Verification items for the finished model (mm, model axes). A direction names the side the tool comes from. Round coordinates to 2 decimals unless told otherwise and drop trailing zeros. Order: outer loops, then holes, each group sorted by start corner. A loop starts at its lowest first (then second) coordinate and runs counter-clockwise, first axis right, second up. Notation, with made-up numbers: (70.5, 73) -> (99.5, 73) arc R26 ccw to (99.5, 95) -> close; hole circle Ø8 at (-2, -28.5). An arc over 180 degrees is marked (long way). Return JSON: item names as keys, results as strings. Group by question number.
1) Section check C-C on x = 0. Enter the section's corners in (y, z).
2) Section check A-A on y = 0. Enter the section's corners in (x, z), plus the area to 3 significant figures.
3) Depth check by flat-ended pin: pin 1 (0.7 mm diameter, centred on x = 0, y = 1, fed in from -Z); pin 2 (0.5 mm diameter, centred on y = 0.5, z = 0.5, fed in from +X). Enter the tip coordinate at first touch or a pass-through.
4) Section check B-B on z = 1.2. Enter the section's corners in (x, y), plus the area to 3 significant figures.
5) Section check D-D on z = 3.95. Enter the section's corners in (x, y).
6) Scan lines: L1, parallel to Y at x = -1.4, z = 1.45; L2, parallel to Y at x = -0.45, z = 2.7; L3, parallel to X at y = -0.4, z = 0.6. Record each from-to range of solid material in increasing order.
7) Tool access check on faces 4 (the flat face through (-0.444, 0, 1)), 5 (the flat face through (1, 0, 0)). Record the directions out of +Z, -Z, +X, -X, +Y, -Y that give a thin tool (end or side, any length) a straight path to the whole face; none if there is none.
8) Draft check along X on faces 1 (the cylindrical face through (1.008, -1.938, 2.317)), 2 (the flat face through (-1, 0, 0)), 3 (the flat face through (0, 0, 1.524)). Enter one of: pulls with the +X half, pulls with the -X half, needs draft (parallel to the pull), parting line crosses it, or undercut.
```python
from build123d import *

# Parameters (mm, degrees)
F0_R     = 2.1844
F1_DEPTH = 5.207
F2_W     = 0.889
F2_H     = 3.048
F3_DEPTH = 12.7
F4_SIZE  = 0.508


with BuildPart() as f1:
    # F0 (on Top) → F1 (new body)
    with BuildSketch(Plane.XY):
        Circle(F0_R)
    extrude(amount=F1_DEPTH)

    # F2 (on Front) → F3 (cut, symmetric)
    with BuildSketch(Plane.XZ):
        Rectangle(F2_W, F2_H)
    extrude(amount=F3_DEPTH, both=True, mode=Mode.SUBTRACT)

    # F4
    f4_edges = [f1.edges().sort_by_distance(p)[0] for p in [
        (-2.1844, 0, 5.207),
    ]]
    chamfer(f4_edges, length=F4_SIZE)


solid = f1.part
```
Check result:
{
 "1": {"outline": "(-2.18, 1.52) -> (2.18, 1.52) -> (2.18, 4.7) -> (1.68, 5.21) -> (-1.68, 5.21) -> (-2.18, 4.7) -> close"},
 "2": {"outline": "(-2.18, 0) -> (-0.44, 0) -> (-0.44, 1.52) -> (0.44, 1.52) -> (0.44, 0) -> (2.18, 0) -> (2.18, 4.7) -> (1.68, 5.21) -> (-1.68, 5.21) -> (-2.18, 4.7) -> close", "area": "21.1 mm^2"},
 "3": {"pin 1": "z = 1.52", "pin 2": "x = 2.17"},
 "4": {"outline": "(-0.44, -2.14) -> (-0.44, 2.14) arc R2.18 ccw to start; (0.44, -2.14) arc R2.18 ccw to (0.44, 2.14) -> close", "area": "11.1 mm^2"},
 "5": {"outline": "circle Ø4.37 at (0, 0)"},
 "6": {"L1": "-1.68 to 1.68", "L2": "-2.14 to 2.14", "L3": "-2.15 to -0.44, 0.44 to 2.15"},
 "7": {"face 4": "-Z, +Y, -Y", "face 5": "-Z, +X, -X, +Y, -Y"},
 "8": {"face 1": "parting line crosses it", "face 2": "needs draft", "face 3": "undercut"}
}
